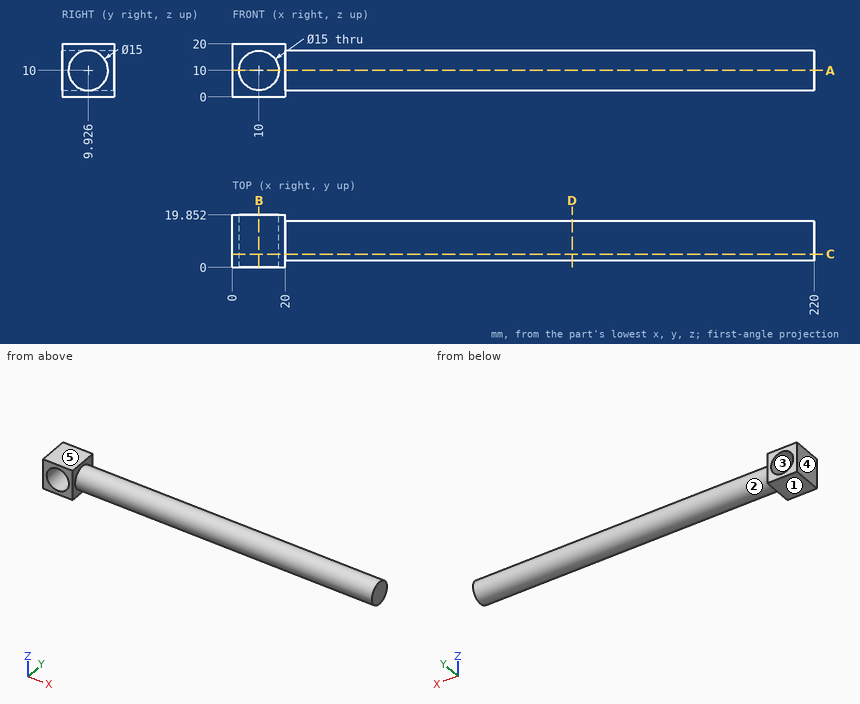
Study the drawing (mm; zero at the part's minimum x, y, z) and answer. A direction names the side the tool comes from. Give positions to 0.01 mm unless a question says otherwise; leave off trailing zeros. Write each loop counter-clockwise with the first axis right and the second up, starting at its lowest first coordinate (ties: lowest second). Pieces come first, ordered by that corner, then holes. Notation, with made-up numbers: (2.5, 86.25) -> (11.5, 86.25) arc R11 ccw to (11.5, 95.25) -> close; hole circle Ø10 at (62, -22). An arc over 180 degrees is marked (long way). Answer as a JSON object with one key per item and string values. Group by question number.
1) Each of these flat-tipped pins is pushed along its axis until it touches: P1, Ø1, axis at x = 193.5, z = 9, coming from the +Y side; P2, Ø10, axis at x = 164.5, y = 2.5, coming from the -Z side; P3, Ø6, axis at x = 154, y = 11, coming from the +Z side. Where does it stop, or does it pass through?
2) A tool of negligible diameter and unlimited length cuts with its end or side. For the marked faces 1 and 2, from which of +Z, -Z, +X, -X, +Y, -Y can it reach the whole face along a straight path? Write none if from no direction.
3) Find section C-C (y = 5). Write down the section's boundary in (x, z), and give its area (3 significant figures).
4) Consider L1, parallel to X at y = 4.5, z = 10; L2, parallel to Y at x = 172, z = 10.75; L3, parallel to X at y = 17, z = 5.25. Determine where each line is inside the solid, lowest interval first. Write a range as from..to.
5) Find section A-A (z = 10). Write down the section's boundary in (x, y).
6) Find section B-B (x = 10). Write down the section's boundary in (y, z).
7) Find section D-D (x = 128.5). Write down the section's boundary in (y, z).
8) The mould has two halves that part along X. Classify the marked faces 3, 4 and 5: +X half, -X half, draft (parallel to the pull), parting line (faces both ways), or undercut.
Values follow:
{
 "1": {"P1": "stops at y = 17.41", "P2": "stops at z = 2.9", "P3": "stops at z = 17.5"},
 "2": {"face 1": "-Z, +X, -X, +Y, -Y", "face 2": "+X"},
 "3": {"outline": "(0, 0) -> (20, 0) -> (20, 4.34) -> (220, 4.34) -> (220, 15.66) -> (20, 15.66) -> (20, 20) -> (0, 20) -> close; hole circle Ø15 at (10, 10)", "area": "2,490 mm2"},
 "4": {"L1": "x = 0..2.5, 17.5..220", "L2": "y = 2.46..17.39", "L3": "x = 0..4.2, 15.8..20"},
 "5": {"outline": "(0, 0) -> (2.5, 0) -> (2.5, 19.85) -> (0, 19.85) -> close; (17.5, 0) -> (20, 0) -> (20, 2.43) -> (220, 2.43) -> (220, 17.43) -> (20, 17.43) -> (20, 19.85) -> (17.5, 19.85) -> close"},
 "6": {"outline": "(0, 0) -> (19.85, 0) -> (19.85, 2.5) -> (0, 2.5) -> close; (0, 17.5) -> (19.85, 17.5) -> (19.85, 20) -> (0, 20) -> close"},
 "7": {"outline": "circle Ø15 at (9.93, 10)"},
 "8": {"face 3": "undercut", "face 4": "-X half", "face 5": "draft"}
}
